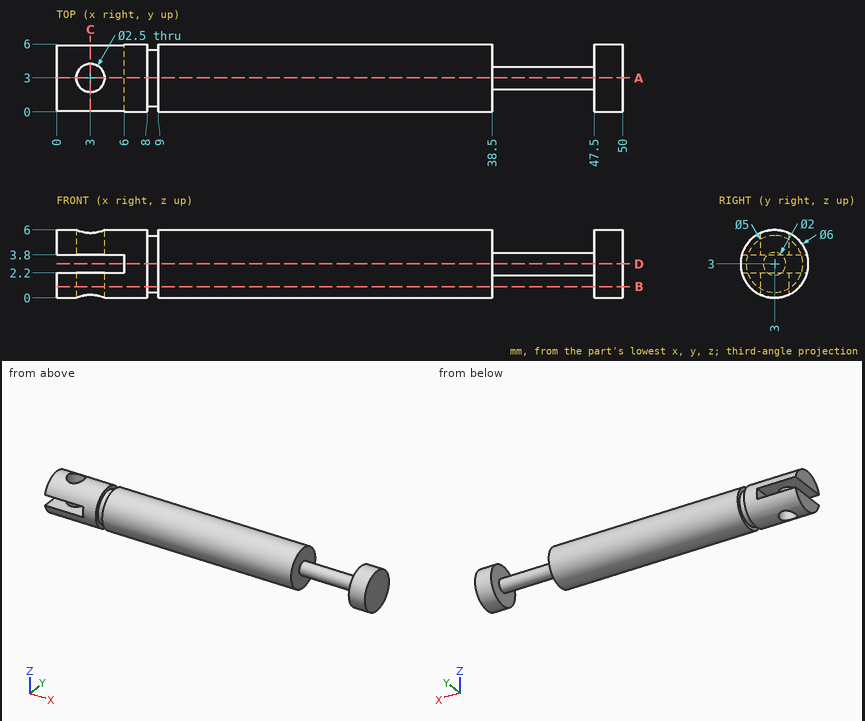
Drawing for the job (mm, zero at the part's lowest x, y, z). Coordinates: 2 decimals unless noted, no trailing zeros. Order: outer loops, then holes, each group sorted by start corner. A loop starts at its lowest first (then second) coordinate and runs counter-clockwise, first axis right, second up. Notation, with made-up numbers: (-34.75, 75.25) - (-8.75, 75.25) arc R15 ccw to (-8.75, 97.25) - close; hole circle Ø3 at (-20, -36). An arc over 180 degrees is marked (long way). Use a Markdown table: item, result. Add a question column.
(1) Flat gauge pins, fed straight in: pin 1 (3 mm diameter, centred on x = 23, y = 1, fed in from +Z); pin 2 (1.5 mm diameter, centred on x = 20.5, z = 0.5, fed in from -Y); pin 3 (0.5 mm diameter, centred on y = 4.5, z = 3, fed in from -X). Where does each tip first touch, or does it go through?
(2) Saw through at D-D (z = 3). Give the cut face in (x, y).
(3) Saw through at C-C (x = 3). Give the cut face in (y, z).
(4) Drill centre lines: line 1 along X through (y, z) = (2.5, 1); line 2 along X through (y, z) = (4, 0.5); line 3 along X through (y, z) = (3.25, 4). Where is each one in solid material? Low to high. Write a range as [from, to].
(5) Saw through at A-A (y = 3). Count the separate pieces of the cut face and the enclosed holes in it, then the cut area to 3 significant figures.
(6) Saw through at B-B (z = 1). Give the cut face in (x, y), then the cut area to 3 significant figures.
Solved:
| question | item | result |
|---|---|---|
| 1 | pin 1 | stops at z = 5.96 |
| 1 | pin 2 | stops at y = 0.56 |
| 1 | pin 3 | stops at x = 6 |
| 2 | outline | (6, 0) - (8, 0) - (8, 0.5) - (9, 0.5) - (9, 0) - (38.5, 0) - (38.5, 2) - (47.5, 2) - (47.5, 0) - (50, 0) - (50, 6) - (47.5, 6) - (47.5, 4) - (38.5, 4) - (38.5, 6) - (9, 6) - (9, 5.5) - (8, 5.5) - (8, 6) - (6, 6) - close |
| 3 | outline | (0.11, 2.2) arc R3 ccw to (1.75, 0.27) - (1.75, 2.2) - close; (0.11, 3.8) - (1.75, 3.8) - (1.75, 5.73) arc R3 ccw to start; (4.25, 0.27) arc R3 ccw to (5.89, 2.2) - (4.25, 2.2) - close; (4.25, 3.8) - (5.89, 3.8) arc R3 ccw to (4.25, 5.73) - close |
| 4 | line 1 | x = [0, 1.85], [4.15, 38.5], [47.5, 50] |
| 4 | line 2 | x = [0, 2.25], [3.75, 8], [9, 38.5], [47.5, 50] |
| 4 | line 3 | x = [0, 1.78], [4.22, 38.5], [47.5, 50] |
| 5 | separate pieces | 3 |
| 5 | enclosed holes | 0 |
| 5 | area | 242 mm² |
| 6 | outline | (0, 0.76) - (8, 0.76) - (8, 1.5) - (9, 1.5) - (9, 0.76) - (38.5, 0.76) - (38.5, 5.24) - (9, 5.24) - (9, 4.5) - (8, 4.5) - (8, 5.24) - (0, 5.24) - close; (47.5, 0.76) - (50, 0.76) - (50, 5.24) - (47.5, 5.24) - close; hole circle Ø2.5 at (3, 3) |
| 6 | area | 177 mm² |
